Work out the finished part from the listing and answer in its coordinate system (mm). A direction names the side the tool comes from. Give positions to 0.01 mm unless a question says otherwise; leave off trailing zeros. Loops run counter-clockwise (first coordinate to the right, second up) from the corner with the lowest first, then second, coordinate; pieces in that order, holes last. Notation, with made-up numbers: (-23, 84) -> (-16, 84) arc R30 ccw to (-16, 109) -> close; hole circle Ø11 at (-11, -1.75). An arc over 180 degrees is marked (long way). Answer as CSV lines item,"result". Start each with the question number.
1. A tool of negligible diameter and unlimited length cuts with its end or side. For faces 4 (the face through (21.38, 14.301, 0.285)), 5 (the face through (21, 14, 3)), 6 (the face through (0.21, 19.07, 3.03)), 7 (the face through (21.38, 14.301, 5.715)), from which of +Z, -Z, +X, -X, +Y, -Y can it reach the whole face along a straight path? Write none if from no direction.
2. Find section B-B, the plane x = 26.5. Give the vertices of the cut face in (y, z).
3. Find the intervals of material crossed by line 1 along Z through (x, y) = (5.5, -2.1); line 2 along Y through (x, z) = (30.6, 3); line 3 along Z through (x, y) = (26.5, 17.5), in increasing order.
4. Determine the mould class of faces 1 (the face through (31.199, 14.285, 2.972)), 2 (the face through (29.528, 18.586, 3.208)), 3 (the face through (9, 10, 6)) for opening direction Y: +Y half, -Y half, draft (parallel to the pull), parting line (faces both ways), or undercut.
5. Find section A-A, the plane z = 3. Count the separate pieces of the cut face and the enclosed holes in it, and give its area (3 significant figures).
6. Flat-ended cylindrical pins translate along their axes: pin 1 Ø3 at (x, z) = (18, 3.5) entering from -Y; pin 2 Ø0.5 at (y, z) = (17, 4) entering from +X; pin 3 Ø3.5 at (x, z) = (5.5, 3) entering from -Y; pin 4 Ø1.9 at (y, z) = (17, 3) entering from +X. Find the tip coordinate at first contact, or state that the pin passes through.
7. Find section D-D, the plane x = 15. Give the vertices of the cut face in (y, z).
8. Find section C-C, the plane y = 12.25. Give the vertices of the cut face in (x, z), and give its area (3 significant figures).
from build123d import *

# Parameters (mm, degrees)
SKETCH_1_W          = 11
SKETCH_1_H          = 20
EXTRUDE_1_DEPTH     = 6
CUT_EXTRUDE_1_DEPTH = 6
SKETCH_3_R          = 5.5
EXTRUDE_2_DEPTH     = 6
SKETCH_4_W          = 24
SKETCH_4_H          = 6
EXTRUDE_3_DEPTH     = 6
SKETCH_6_R          = 1.5
CUT_EXTRUDE_3_DEPTH = 6
SKETCH_7_R          = 1.5
CUT_EXTRUDE_4_DEPTH = 6
SKETCH_5_W          = 6
SKETCH_5_H          = 0.5
CUT_EXTRUDE_5_DEPTH = 10
SKETCH_15_W         = 6
SKETCH_15_H         = 6
EXTRUDE_4_DEPTH     = 2
FILLET_2_R          = 1
SKETCH_16_R         = 1.6
CUT_EXTRUDE_7_DEPTH = 4
SKETCH_14_R         = 1.6
CUT_EXTRUDE_8_DEPTH = 4


# Read off the part's stored shape, not the designer's step: 切除-拉伸1
with BuildPart() as part:
    # 草图1 → 凸台-拉伸1 (new body)
    with BuildSketch(Plane.XY):
        with Locations((5.5, 10)):
            Rectangle(SKETCH_1_W, SKETCH_1_H)
    extrude(amount=EXTRUDE_1_DEPTH)

    # 切除-拉伸1 outline → 切除-拉伸1 (cut)
    with BuildSketch(Plane.XY):
        with BuildLine():
            Line((0, 20), (0, 19.228884523))
            ThreePointArc((0, 19.228884523), (2.723103392, 19.806282974), (5.5, 20))
            Line((5.5, 20), (0, 20))
        make_face()
        with BuildLine():
            Line((11, 20), (5.5, 20))
            ThreePointArc((5.5, 20), (8.276896608, 19.806282974), (11, 19.228884523))
            Line((11, 19.228884523), (11, 20))
        make_face()
    extrude(amount=CUT_EXTRUDE_1_DEPTH, mode=Mode.SUBTRACT)

    # 草图3 → 凸台-拉伸2 (add)
    with BuildSketch(Plane.XY):
        with Locations((5.5, 0)):
            Circle(SKETCH_3_R)
    extrude(amount=EXTRUDE_2_DEPTH)

    # 草图4 → 凸台-拉伸3 (add)
    with BuildSketch(Plane.XY):
        with Locations((17.5, 17)):
            Rectangle(SKETCH_4_W, SKETCH_4_H)
    extrude(amount=EXTRUDE_3_DEPTH)

    # 草图6 → 切除-拉伸3 (cut)
    with BuildSketch(Plane.XY):
        with Locations((5.5, 0)):
            Circle(SKETCH_6_R)
    extrude(amount=CUT_EXTRUDE_3_DEPTH, mode=Mode.SUBTRACT)

    # 草图7 → 切除-拉伸4 (cut)
    with BuildSketch(Plane.XZ.offset(-14)):
        with Locations((26.5, 3)):
            Circle(SKETCH_7_R)
    extrude(amount=-CUT_EXTRUDE_4_DEPTH, mode=Mode.SUBTRACT)

    # 草图5 → 切除-拉伸5 (cut)
    with BuildSketch(Plane.XY):
        with Locations((5.5, -5.25)):
            Rectangle(SKETCH_5_W, SKETCH_5_H)
    extrude(amount=CUT_EXTRUDE_5_DEPTH, mode=Mode.SUBTRACT)

    # 草图15 → 凸台-拉伸4 (add)
    with BuildSketch(Plane(origin=(29.5, 0, 0), x_dir=(0, 0, -1), z_dir=(1, 0, 0))):
        with Locations((-3, 17)):
            Rectangle(SKETCH_15_W, SKETCH_15_H)
    extrude(amount=EXTRUDE_4_DEPTH)

    # 圆角2
    fillet_2_edges = [part.edges().sort_by_distance(p)[0] for p in [
        (31.5, 17, 0),
        (31.5, 20, 3),
        (31.5, 17, 6),
        (31.5, 14, 3),
        (11, 7, 6),
        (0, 9.614442262, 0),
        (0, 9.614442262, 6),
        (0, 19.228884523, 3),
        (0.871172764, -2.970514841, 0),
        (0.871172764, -2.970514841, 6),
        (2.723103392, 19.806282974, 6),
        (2.723103392, 19.806282974, 0),
        (11, 14, 3),
        (11, 7, 0),
        (21.25, 14, 0),
        (21.25, 14, 6),
        (18.5, 20, 6),
        (18.5, 20, 0),
        (10.128827236, -2.970514841, 6),
        (10.128827236, -2.970514841, 0),
        (7.791287847, -5, 3),
        (3.208712153, -5, 3),
        (5.5, -5, 0),
        (5.5, -5, 6),
    ]]
    fillet(fillet_2_edges, radius=FILLET_2_R)

    # 草图16 → 切除-拉伸7 (cut)
    with BuildSketch(Plane(origin=(31.5, 0, 0), x_dir=(0, 0, -1), z_dir=(1, 0, 0))):
        with Locations((-3, 17)):
            Circle(SKETCH_16_R)
    extrude(amount=-CUT_EXTRUDE_7_DEPTH, mode=Mode.SUBTRACT)

    # 草图14 → 切除-拉伸8 (cut)
    with BuildSketch(Plane(origin=(0, -5, 0), x_dir=(-1, 0, 0), z_dir=(0, -1, 0))):
        with Locations(Location((-5.5, -3, 0), (0, 0, 90))):
            Circle(SKETCH_14_R)
    extrude(amount=-CUT_EXTRUDE_8_DEPTH, mode=Mode.SUBTRACT)


solid = part.part
Resolved:
1,face 4,"-Z, +X, -Y"
1,face 5,"+Z, -Z, +X, -Y"
1,face 6,"+Z, -Z, -X, +Y"
1,face 7,"+Z, +X, -Y"
2,outline,"(14, 1) arc R1 ccw to (15, 0) -> (19, 0) arc R1 ccw to (20, 1) -> (20, 1.5) -> (14, 1.5) -> close; (14, 4.5) -> (20, 4.5) -> (20, 5) arc R1 ccw to (19, 6) -> (15, 6) arc R1 ccw to (14, 5) -> close"
3,line 1,"z = 0 to 1.4, 4.6 to 6"
3,line 2,"y = 14.01 to 15.4, 18.6 to 19.99"
3,line 3,"z = 0 to 1.5, 4.5 to 6"
4,face 1,"-Y half"
4,face 2,"undercut"
4,face 3,"draft"
5,separate pieces,"3"
5,enclosed holes,"0"
5,area,"339 mm^2"
6,pin 1,"stops at y = 14"
6,pin 2,"stops at x = 27.5"
6,pin 3,"stops at y = -5"
6,pin 4,"stops at x = 25.34"
7,outline,"(14, 1) arc R1 ccw to (15, 0) -> (19, 0) arc R1 ccw to (20, 1) -> (20, 5) arc R1 ccw to (19, 6) -> (15, 6) arc R1 ccw to (14, 5) -> close"
8,outline,"(0, 1) arc R1 ccw to (1, 0) -> (10, 0) arc R1 ccw to (11, 1) -> (11, 5) arc R1 ccw to (10, 6) -> (1, 6) arc R1 ccw to (0, 5) -> close"
8,area,"65.1 mm^2"
